Could you check a few things on this model? Use its own coordinates, in mm. Face numbers are marked on the shaded views. A direction names the side the tool comes from. Give positions to 0.01 mm unless a question says otherwise; leave off trailing zeros. Order: outer loops, then holes, each group sorted by start corner. A loop starts at its lowest first (then second) coordinate and runs counter-clockwise, first axis right, second up. Notation, with made-up numbers: (72.5, 42.25) -> (85.5, 42.25) arc R20 ccw to (85.5, 81.25) -> close; hole circle Ø11 at (60, 20). An arc over 180 degrees is marked (long way). Write each question's results on one line, items separated by ' | '.
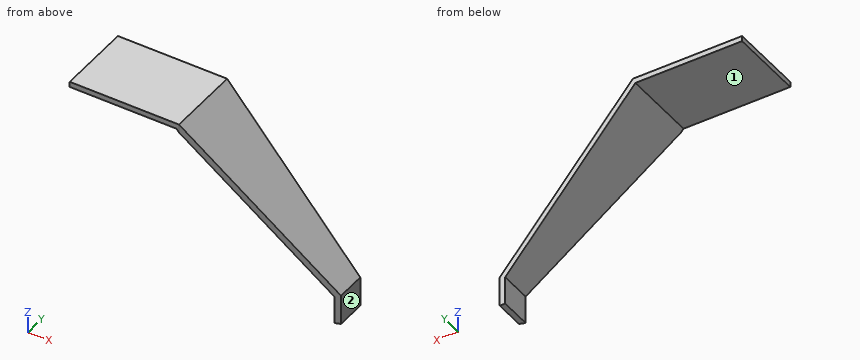
```python
from build123d import *

# Parameters (mm, degrees)
F1_DEPTH = 55
F3_DEPTH = 150


with BuildPart() as f1:
    # F0 (on Front) → F1 (new body)
    with BuildSketch(Plane.XZ):
        Polygon((80, 0), (0, 0), (0, -4), (78.15749, -4), (173.488461, -115.477098), (173.488461, -136), (177.488461, -136), (177.488461, -114), align=None)
    extrude(amount=F1_DEPTH)

    # F2 (on Top) → F3 (cut)
    with BuildSketch(Plane.XY):
        Polygon((177.488461, -22), (80, -55), (177.488461, -55), align=None)
    extrude(amount=-F3_DEPTH, mode=Mode.SUBTRACT)


solid = f1.part
```
Q1. I'm going to push flat-ended pins straight in: pin 1 Ø6 at (x, y) = (126, -12.5) entering from +Z; pin 2 Ø1 at (x, y) = (57, -17.5) entering from -Z; pin 3 Ø2 at (y, z) = (-11.5, -89.5) entering from +X. Where does each tip first touch, or does it pass through?
Here are the results:
pin 1: stops at z = -50.28 | pin 2: stops at z = -4 | pin 3: stops at x = 157.39
Q2. Suppose I cut it at A-A on y = -15.5. Please give me the cut outline in (x, z), and give its area (3 significant figures).
Here are the results:
outline: (0, -4) -> (78.16, -4) -> (173.49, -115.48) -> (173.49, -136) -> (177.49, -136) -> (177.49, -114) -> (80, 0) -> (0, 0) -> close | area: 995 mm²
Q3. Suppose I cut it at B-B on x = 46.5. Please give me the cut outline in (y, z), and give its area (3 significant figures).
Here are the results:
outline: (-55, -4) -> (0, -4) -> (0, 0) -> (-55, 0) -> close | area: 220 mm²
Q4. For the marked faces 1 and 2, which set-ups out of +Z, -Z, +X, -X, +Y, -Y let a thin tool reach every point of the face, with its end or its side?
Here are the results:
face 1: -Z, -X, +Y, -Y | face 2: +Z, -Z, +X, +Y, -Y
Q5. Suppose I cut it at D-D on y = -51. Please give me the cut outline in (x, z).
Here are the results:
outline: (0, -4) -> (78.16, -4) -> (91.82, -19.97) -> (91.82, -13.82) -> (80, 0) -> (0, 0) -> close
Q6. Suppose I cut it at C-C on z = -74. Please give me the cut outline in (x, y), and give its area (3 significant figures).
Here are the results:
outline: (138.02, -35.36) -> (143.28, -33.58) -> (143.28, 0) -> (138.02, 0) -> close | area: 181 mm²
Q7. I need wall thicknesses on line 1 along Z through (x, y) = (20.5, -14); line 2 along Z through (x, y) = (87, -10); line 3 along X through (y, z) = (-24, -14.5). Which ranges of each line are inside material? Lowest first, please.
Here are the results:
line 1: z = -4 to 0 | line 2: z = -14.34 to -8.19 | line 3: x = 87.14 to 92.4
